from build123d import *

# Parameters (mm, degrees)
PAD_DEPTH    = 40
POCKET_DEPTH = 39


with BuildPart() as part:
    # Sketch → Pad (new body)
    with BuildSketch(Plane.XY):
        with BuildLine():
            ThreePointArc((0, -37), (34.183543, 14.159287), (-26.162951, 26.162951))
            Line((-22.627417, 22.627417), (-26.162951, 26.162951))
            ThreePointArc((0, -32), (29.564145, 12.24587), (-22.627417, 22.627417))
            Line((0, -37), (0, -32))
        make_face()
    extrude(amount=PAD_DEPTH)

    # Sketch001 → Pocket (cut)
    with BuildSketch(Plane.XY.offset(40)):
        Polygon((0, 0), (-30.679579, 37.886125), (-2.393788, 45.676197), align=None)
        Polygon((0, 0), (2.341637, 44.681104), (37.049321, 41.14744), align=None)
        Polygon((0, 0), (39.999108, 36.015358), (48.030265, 2.51716), align=None)
        Polygon((0, 0), (49.461223, -2.592153), (39.264005, -35.353469), align=None)
        Polygon((0, 0), (33.741126, -37.473316), (4.909112, -46.707078), align=None)
    extrude(amount=-POCKET_DEPTH, mode=Mode.SUBTRACT)


solid = part.part
Read the model definition and answer for the solid it produces. Units are mm, in the model's axes. A direction names the side the tool comes from. Give positions to 0.01 mm unless a question says otherwise; leave off trailing zeros. Write each loop counter-clockwise with the first axis right and the second up, starting at its lowest first coordinate (ties: lowest second). Pieces come first, ordered by that corner, then holes. Notation, with made-up numbers: M 48,49.5 L 66,49.5 A36 cw 66,88.5 Z; hole C -37,-32 d11. An arc over 180 degrees is marked long. One line per item, written item: value. Start each with the question number.
(1) Find the intervals of material crossed by line 1 (X direction, y = 0, z = 8.5); line 2 (Y direction, x = 23, z = 11.5); line 3 (Z direction, x = 15.5, y = 28.5), in increasing order.
(2) A tool of negligible diameter and unlimited length cuts with its end or side. For faces 1 (the flat face through (34.488, 1.807, 20.773)), 2 (the flat face through (3.61, -34.35, 20.77)), 3 (the flat face through (25.665, -23.108, 20.773)), 4 (the flat face through (34.418, -1.804, 20.773)), 5 (the flat face through (23.108, 25.665, 20.773)), from which of +Z, -Z, +X, -X, +Y, -Y can it reach the whole face along a straight path? Write none if from no direction.
(3) Find section D-D (y = 0). Determine the outline of the cut face in (x, z), plus the area to 3 significant figures.
(4) Find section A-A (z = 18). Determine the outline of the cut face in (x, y).
(5) Find section B-B (x = 9). Determine the outline of the cut face in (y, z), plus the area to 3 significant figures.
(6) Flat-ended cylindrical pins translate along their axes: pin 1 Ø14.5 at (x, y) = (31, 13) entering from +Z; pin 2 Ø5.5 at (y, z) = (-34.5, 21.5) entering from -X; pin 3 Ø3 at (x, z) = (30.5, 28.5) entering from +Y. Find the tip coordinate at first contact, or state that the pin passes through.
(7) Determine the mould class of faces 6 (the flat face through (24, -24, 40)), 7 (the flat face through (25.61, 23.06, 20.77)), 8 (the flat face through (-21.7, 26.8, 20.8)), 9 (the cylindrical face through (21.834, 23.394, 18.425)) for opening direction X: pulls with the +X half, pulls with the -X half, needs draft (parallel to the pull), parting line crosses it, or undercut.
(8) Find section C-C (x = 30). Determine the outline of the cut face in (y, z).
Results below:
1. line 1: x = 32 to 37
1. line 2: y = -25.54 to -22.25, 22.25 to 25.54
1. line 3: z = 0 to 1
2. face 1: +Z, -X, +Y
2. face 2: +Z, +X, +Y
2. face 3: +Z, +X
2. face 4: +Z, -X, -Y
2. face 5: +Z, +Y
3. outline: M 32,0 L 37,0 L 37,40 L 32,40 Z
3. area: 200 mm^2
4. outline: M -26.16,26.16 L -22.63,22.63 A32 cw -20.14,24.87 L -23.28,28.75 A37 ccw Z; M -1.94,36.95 L -1.67,31.96 A32 cw 1.67,31.96 L 1.94,36.95 A37 ccw Z; M 0,-37 A37 ccw 3.87,-36.8 L 3.34,-31.82 A32 cw 0,-32 Z; M 21.41,-23.78 L 24.76,-27.5 A37 ccw 27.5,-24.76 L 23.78,-21.41 A32 cw Z; M 21.41,23.78 A32 cw 23.78,21.41 L 27.5,24.76 A37 ccw 24.76,27.5 Z; M 31.96,-1.67 L 36.95,-1.94 A37 ccw 36.95,1.94 L 31.96,1.67 A32 cw Z
5. outline: M -35.89,0 L -30.71,0 L -30.71,1 L -35.89,1 Z; M 30.71,0 L 35.89,0 L 35.89,1 L 30.71,1 Z
5. area: 10.4 mm^2
6. pin 1: stops at z = 1
6. pin 2: stops at x = 0
6. pin 3: stops at y = 1.68
7. face 6: needs draft
7. face 7: pulls with the +X half
7. face 8: undercut
7. face 9: undercut
8. outline: M -21.66,0 L -11.14,0 L -11.14,1 L -21.66,1 Z; M 11.14,0 L 21.66,0 L 21.66,1 L 11.14,1 Z
